Can you work these out from the model? Positions are in its coordinate system, mm. Face numbers are marked on the shaded views. A direction names the side the tool comes from. Coordinates: 2 decimals unless noted, no trailing zeros. Write each loop counter-clockwise with the first axis right and the second up, starting at its lowest first coordinate (ties: lowest second). Pieces come first, ordered by that corner, then holes. Notation, with made-up numbers: M 31,1.25 L 43,1.25 A19 cw 43,9.25 Z; hole C 55,44.5 d1. An arc over 180 degrees is marked long. Use one line per item in the form item = value. Start each with the question number.
```python
from build123d import *

# Parameters (mm, degrees)
F1_DEPTH = 63.5
F0_W     = 25.4
F0_H     = 19.05
F2_DEPTH = 25.4
F3_DEPTH = 15.875


with BuildPart() as f1:
    # F0 (on Front) → F1 (new body, symmetric)
    with BuildSketch(Plane.XZ):
        Polygon((41.275, -9.525), (41.275, 9.525), (22.225, 9.525), (-41.275, 9.525), (-41.275, -9.525), align=None)
    extrude(amount=F1_DEPTH, both=True)

    # F0 (on Front) → F2 (join, symmetric)
    with BuildSketch(Plane.XZ):
        with BuildLine():
            Line((22.225, 9.525), (41.275, 9.525))
            Line((41.275, 9.525), (41.275, 27.0002))
            ThreePointArc((41.275, 27.0002), (45.9246798487, 38.2255201513), (57.15, 42.8752))
            Line((57.15, 42.8752), (60.325, 42.8752))
            Line((60.325, 42.8752), (60.325, 61.9252))
            Line((60.325, 61.9252), (57.15, 61.9252))
            ThreePointArc((57.15, 61.9252), (32.4542956671, 51.6959043329), (22.225, 27.0002))
            Line((22.225, 27.0002), (22.225, 9.525))
        make_face()
        with Locations((73.025, 52.4002)):
            Rectangle(F0_W, F0_H)
    extrude(amount=F2_DEPTH, both=True)

    # F0 (on Front) → F3 (join)
    with BuildSketch(Plane.XZ):
        with BuildLine():
            Line((-41.275, 9.525), (22.225, 9.525))
            Line((22.225, 9.525), (22.225, 27.0002))
            ThreePointArc((22.225, 27.0002), (32.4542956671, 51.6959043329), (57.15, 61.9252))
            add(Edge.make_bspline(
                [(-41.275, 9.525), (-41.0052500665, 37.4122597277), (10.2264313027, 61.962634325), (57.15, 61.9252)],
                knots=[0, 0, 0, 0, 111.5045361635, 111.5045361635, 111.5045361635, 111.5045361635], degree=3))
        make_face()
    extrude(amount=F3_DEPTH)

    # F0 (on Front) → F4 (revolve)
    with BuildSketch(Plane.XZ):
        Polygon((85.725, 61.9252), (85.725, 42.8752), (85.725, 38.1), (111.125, 38.1), (111.125, 66.675), (85.725, 66.675), align=None)
    revolve(axis=Axis((85.725, 0, 52.3875), (0, 0, 1)))


solid = f1.part
```
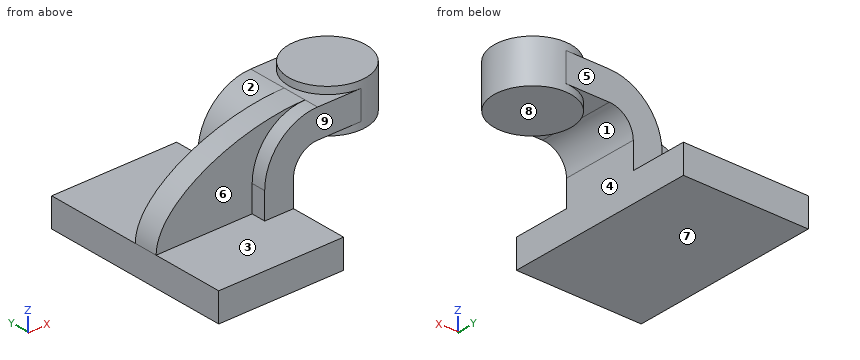
1) Suppose I cut it at B-B on x = 88. Please give me the cut outline in (y, z) (3 decimals).
2) Please list where these lines run through material, in increasing order: line 1 (Z direction, x = 29.5, y = -41) (3 decimals); line 2 (X direction, y = -1.5, z = 39); line 3 (X direction, y = -58, z = 3.5) (3 decimals).
3) Suppose I cut it at C-C on y = 22.5. Please give me the cut outline in (x, z) (3 decimals).
4) Will these pins go through, and if not, where does the flat tip stop? pin 1 Ø2 at (y, z) = (18.5, 56.5) entering from -X; pin 2 Ø15.5 at (x, z) = (-16.5, 36.5) entering from +Y; pin 3 Ø8.5 at (x, y) = (69.5, 2) entering from -Z.
5) If we mould it in two halves opening along X, with no side actions, what happens to the marked faces 1, 2, 3 and 4? For each: +X half, -X half, draft (parallel to the pull), parting line (faces both ways), or undercut.
6) Suppose I cut it at A-A on y = 4.5. Please give me the cut outline in (x, z) (3 decimals), and give its area (3 significant figures).
7) Which directions (+Z, -Z, +X, -X, +Y, -Y) give clear straight access to the entire face, cutting with the end or side of a thin tool? Please do the marked faces 5, 6, 7, 8 and 9.
8) Suppose I cut it at D-D on y = -48.5. Please give me the cut outline in (x, z) (3 decimals).
Computed values:
q1.outline = M -25.298,38.1 L 25.298,38.1 L 25.298,66.675 L -25.298,66.675 Z
q2.line_1 = -9.525 to 9.525
q2.line_2 = -21.51 to 46.76, 60.37 to 111.08
q2.line_3 = -41.275 to 41.275
q3.outline = M -41.275,-9.525 L 41.275,-9.525 L 41.275,27 A15.875 cw 57.15,42.875 L 73.939,42.875 L 73.939,38.1 L 97.511,38.1 L 97.511,66.675 L 73.939,66.675 L 73.939,61.925 L 57.15,61.925 A34.925 ccw 22.225,27 L 22.225,9.525 L -41.275,9.525 Z
q4.pin_1 = 36.96
q4.pin_2 = 0
q4.pin_3 = 38.1
q5.face_1 = undercut
q5.face_2 = -X half
q5.face_3 = draft
q5.face_4 = +X half
q6.outline = M -41.275,-9.525 L 41.275,-9.525 L 41.275,27 A15.875 cw 57.15,42.875 L 60.727,42.875 L 60.727,38.1 L 110.723,38.1 L 110.723,66.675 L 60.727,66.675 L 60.727,61.925 L 57.15,61.925 A34.925 ccw 22.225,27 L 22.225,9.525 L -41.275,9.525 Z
q6.area = 4,160 mm²
q7.face_5 = +Z, +X, -X, +Y
q7.face_6 = +Z, -X, -Y
q7.face_7 = -Z, +X, -X, +Y, -Y
q7.face_8 = -Z, +X, +Y, -Y
q7.face_9 = +Z, +X, -X, -Y
q8.outline = M -41.275,-9.525 L 41.275,-9.525 L 41.275,9.525 L -41.275,9.525 Z
